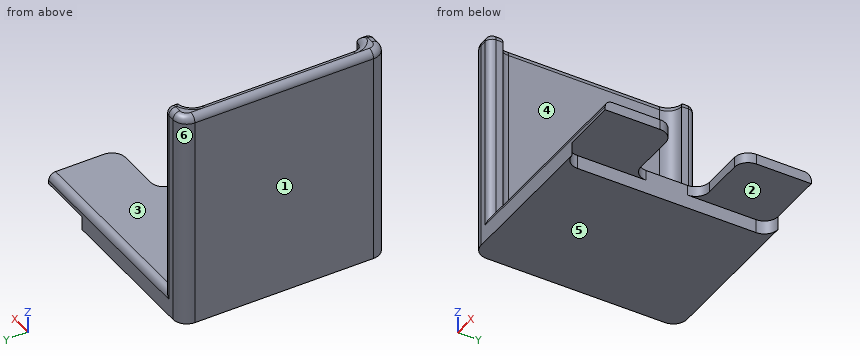
from build123d import *

# Parameters (mm, degrees)
BOSS_EXTRUDE1_DEPTH = 7.5
BOSS_EXTRUDE2_DEPTH = 150
BOSS_EXTRUDE3_START = -10
BOSS_EXTRUDE3_DEPTH = 10
FILLET1_R           = 5
FILLET2_R           = 10
FILLET3_R           = 10


with BuildPart() as part:
    # Sketch1 → Boss-Extrude1 (new body)
    with BuildSketch(Plane.XY):
        with BuildLine():
            Line((-40, 75), (-40, 65))
            ThreePointArc((-40, 65), (-47.071067812, 62.071067812), (-50, 55))
            Line((-50, 55), (-50, -55))
            ThreePointArc((-50, -55), (-47.071067812, -62.071067812), (-40, -65))
            Line((-40, -65), (-40, -75))
            Line((-40, -75), (100, -75))
            Line((100, -75), (100, -25))
            Line((100, -25), (50, -25))
            Line((50, -25), (50, 25))
            Line((50, 25), (100, 25))
            Line((100, 25), (100, 75))
            Line((100, 75), (-40, 75))
        make_face()
    extrude(amount=BOSS_EXTRUDE1_DEPTH)

    # Sketch1<5> → Boss-Extrude2 (add)
    with BuildSketch(Plane.XY):
        with BuildLine():
            ThreePointArc((-50, 55), (-47.071067812, 62.071067812), (-40, 65))
            Line((-40, 65), (-40, 75))
            Line((-40, 75), (-50, 75))
            ThreePointArc((-50, 75), (-57.071067812, 72.071067812), (-60, 65))
            Line((-60, 65), (-60, -65))
            ThreePointArc((-60, -65), (-57.071067812, -72.071067812), (-50, -75))
            Line((-50, -75), (-40, -75))
            Line((-40, -75), (-40, -65))
            ThreePointArc((-40, -65), (-47.071067812, -62.071067812), (-50, -55))
            Line((-50, -55), (-50, 55))
        make_face()
    extrude(amount=BOSS_EXTRUDE2_DEPTH)

    # Sketch1<6> → Boss-Extrude3 (add)
    with BuildSketch(Plane.XY.offset(BOSS_EXTRUDE3_START)):
        with BuildLine():
            Line((-50, -75), (60, -75))
            ThreePointArc((60, -75), (52.928932188, -72.071067812), (50, -65))
            Line((50, -65), (50, 65))
            ThreePointArc((50, 65), (52.928932188, 72.071067812), (60, 75))
            Line((60, 75), (-50, 75))
            ThreePointArc((-50, 75), (-57.071067812, 72.071067812), (-60, 65))
            Line((-60, 65), (-60, -65))
            ThreePointArc((-60, -65), (-57.071067812, -72.071067812), (-50, -75))
        make_face()
    extrude(amount=BOSS_EXTRUDE3_DEPTH)

    # Fillet1
    fillet1_edges = [part.edges().sort_by_distance(p)[0] for p in [
        (30, 75, 7.5),
        (-57.071067812, -72.071067812, 150),
        (30, -75, 7.5),
        (-40, -75, 78.75),
        (-40, -70, 150),
        (-47.071067812, -62.071067812, 150),
        (-45, 75, 150),
        (-40, 75, 78.75),
        (-57.071067812, 72.071067812, 150),
        (-60, 0, 150),
        (-45, -75, 150),
        (-50, 0, 150),
        (-47.071067812, 62.071067812, 150),
        (-40, 70, 150),
    ]]
    fillet(fillet1_edges, radius=FILLET1_R - 0.0001)  # a hair under: the kernel refuses the full size

    # Fillet2
    fillet2_edges = [part.edges().sort_by_distance(p)[0] for p in [
        (100, 25, 3.75),
        (100, -25, 3.75),
    ]]
    fillet(fillet2_edges, radius=FILLET2_R)

    # Fillet3
    fillet3_edges = [part.edges().sort_by_distance(p)[0] for p in [
        (50, 25, 3.75),
        (50, -25, 3.75),
    ]]
    fillet(fillet3_edges, radius=FILLET3_R)


solid = part.part
For this review, take the finished solid that the model builds, in its own axes (mm). Face numbers are marked on the shaded views. A direction names the side the tool comes from. Round coordinates to 2 decimals unless told otherwise and drop trailing zeros. Loops run counter-clockwise (first coordinate to the right, second up) from the corner with the lowest first, then second, coordinate; pieces in that order, holes last. Notation, with made-up numbers: (9, -7) - (62, -7) arc R34 cw to (62, 32) - close; hole circle Ø6 at (83, 66). An arc over 180 degrees is marked (long way). Answer as CSV lines item,"result".
(1) Consider section B-B on z = 42. Give the boundary of the cut face in (x, y), then the cut area to 3 significant figures.
Checked values:
outline,"(-60, -65) arc R10 ccw to (-50, -75) - (-45, -75) arc R5 ccw to (-40, -70) - (-40, -65) arc R10 cw to (-50, -55) - (-50, 55) arc R10 cw to (-40, 65) - (-40, 70) arc R5 ccw to (-45, 75) - (-50, 75) arc R10 ccw to (-60, 65) - close"
area,"1,690 mm2"
(2) Consider section A-A on x = 82.5. Give the boundary of the cut face in (y, z).
Checked values:
outline,"(-75, 0) - (-25, 0) - (-25, 7.5) - (-70, 7.5) arc R5 ccw to (-75, 2.5) - close; (25, 0) - (75, 0) - (75, 2.5) arc R5 ccw to (70, 7.5) - (25, 7.5) - close"
(3) Consider section D-D on x = -12.5. Give the boundary of the cut face in (y, z), then the cut area to 3 significant figures.
Checked values:
outline,"(-75, -10) - (75, -10) - (75, 2.5) arc R5 ccw to (70, 7.5) - (-70, 7.5) arc R5 ccw to (-75, 2.5) - close"
area,"2,610 mm2"
(4) Tool access review of the marked faces 1, 2 and 3: name each direction out of +Z, -Z, +X, -X, +Y, -Y from which nothing blocks a thin tool from reaching the whole face with its end or side.
Checked values:
face 1,"+Z, -Z, -X, +Y, -Y"
face 2,"-Z, +X"
face 3,"+Z, +X"
(5) Insertion check: P1, Ø2, axis at x = -27.5, y = -49.5, coming from the +Z side; P2, Ø5, axis at x = 82.5, y = -51.5, coming from the -Z side; P3, Ø4, axis at y = 67.5, z = 64, coming from the +X side. Each pin has a flat end and moves straight along its axis. Give the tip position at first contact, or say it passes through.
Checked values:
P1,"stops at z = 7.5"
P2,"stops at z = 0"
P3,"stops at x = -40"
(6) Mouldability with a two-part tool opening along Y and no side actions: class the marked faces 4, 5 and 6 as +Y half, -Y half, draft (parallel to the pull), parting line (faces both ways), or undercut.
Checked values:
face 4,"undercut"
face 5,"draft"
face 6,"+Y half"
(7) Wall thickness on line 1 (Z direction, x = 6, y = -66.5); line 2 (X direction, y = -52, z = 57); line 3 (Z direction, x = 72, y = -38.5): over which ranges is each line inside the solid? List them lowest first.
Checked values:
line 1,"z = -10 to 7.5"
line 2,"x = -60 to -50"
line 3,"z = 0 to 7.5"
